Could you check a few things on this drawing? It's one solid part, dimensions in mm from its lowest x, y, z. Give positions to 0.01 mm unless a question says otherwise; leave off trailing zeros. Loops run counter-clockwise (first coordinate to the right, second up) from the corner with the lowest first, then second, coordinate; pieces in that order, holes last. Notation, with made-up numbers: (20.25, 50) -> (69.25, 50) arc R21 cw to (69.25, 74) -> close; hole circle Ø10 at (87, 71.5). An arc over 180 degrees is marked (long way). Use CSV: the item, a comma, the result in double quotes.
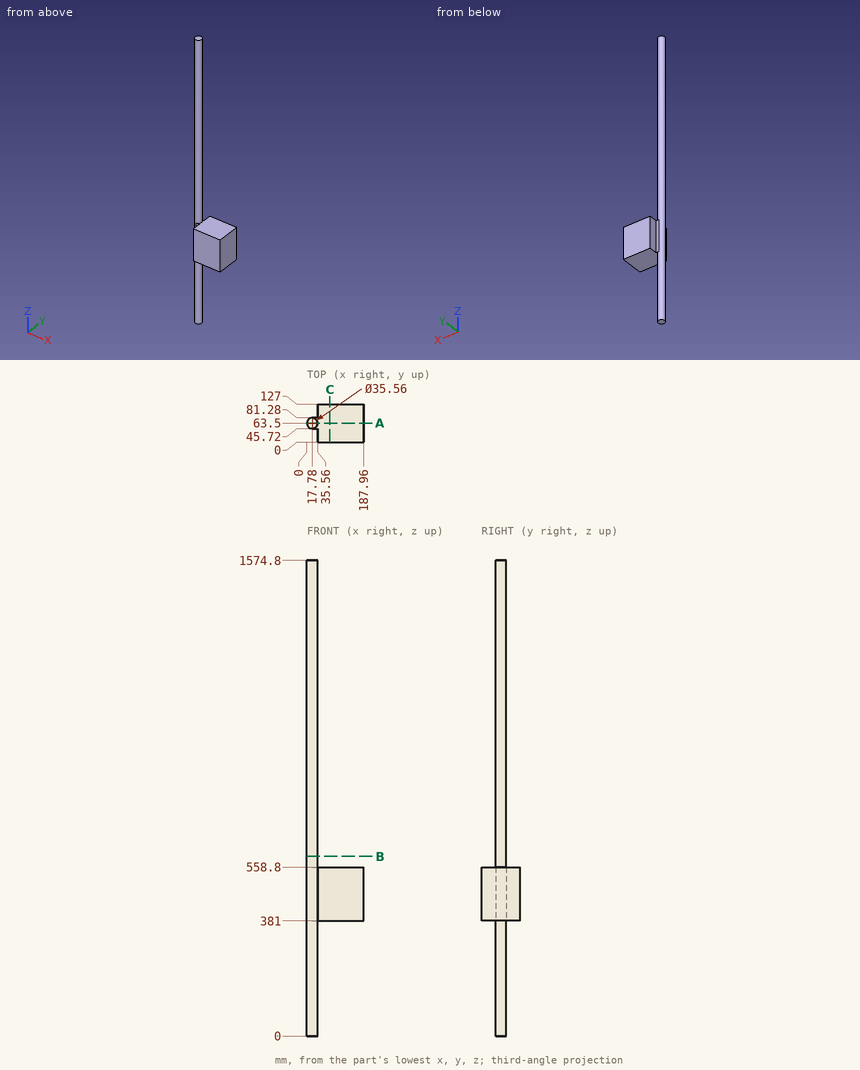
(1) Will these pins go through, and if not, where does the flat tip stop? pin 1 Ø1.5 at (x, y) = (48, 82.5) entering from -Z; pin 2 Ø14 at (x, z) = (24.5, 431.5) entering from +Y; pin 3 Ø1.5 at (x, z) = (34.5, 205) entering from -Y.
Answer sheet:
pin 1,"stops at z = 381"
pin 2,"stops at y = 81.28"
pin 3,"stops at y = 55.68"
(2) If we section it at B-B, the plane z = 595: Write out the boundary of the cut face in (x, y), then the cut area to 3 significant figures.
Answer sheet:
outline,"circle Ø35.56 at (17.78, 63.5)"
area,"993 mm2"
(3) If I drill on L1, parallel to Z at x = 49.5, y = 113; L2, parallel to Y at x = 22.5, z = 1221; L3, parallel to Y at x = 21.5, z = 1289, over which ranges is the centre line in solid material (lowest first)? Write a range as from..to.
Answer sheet:
L1,"z = 381..558.8"
L2,"y = 46.36..80.64"
L3,"y = 46.11..80.89"
(4) If we section it at A-A, the plane y = 63.5: Write out the boundary of the cut face in (x, z), then the cut area to 3 significant figures.
Answer sheet:
outline,"(0, 0) -> (35.56, 0) -> (35.56, 381) -> (187.96, 381) -> (187.96, 558.8) -> (35.56, 558.8) -> (35.56, 1574.8) -> (0, 1574.8) -> close"
area,"83,100 mm2"
(5) If we section it at C-C, the plane x = 76: Write out the boundary of the cut face in (y, z), then the cut area to 3 significant figures.
Answer sheet:
outline,"(0, 381) -> (127, 381) -> (127, 558.8) -> (0, 558.8) -> close"
area,"22,600 mm2"
